For this review, take the finished solid that the model builds, in its own axes (mm). Face numbers are marked on the shaded views. Coordinates: 2 decimals unless noted, no trailing zeros. Write each question's results on one line, items separated by ' | '.
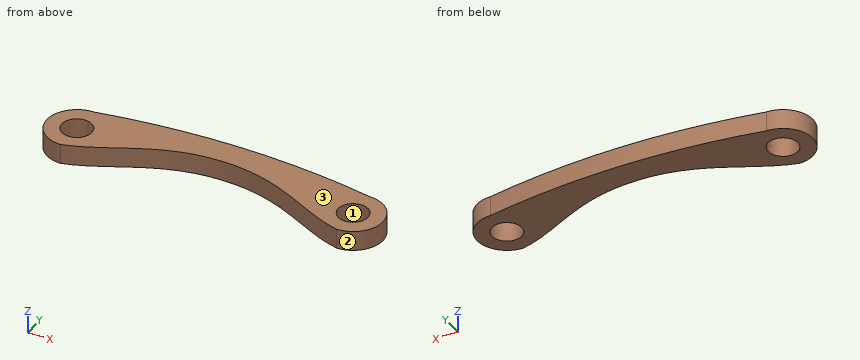
from build123d import *

# Parameters (mm, degrees)
SKETCH1_R           = 1.5
BOSS_EXTRUDE1_DEPTH = 2


with BuildPart() as part:
    # Sketch1 → Boss-Extrude1 (new body)
    with BuildSketch(Plane.XY):
        with BuildLine():
            ThreePointArc((-14, 3), (-17, 0), (-14, -3))
            add(Edge.make_bspline(
                [(-14, -3), (-10.110775288, -2.025488943), (-6.332313911, 1.681383892), (6.35903931, 1.579555666), (10.137986604, -2.11235599), (14, -3)],
                knots=[0, 0, 0, 0, 0.449202302, 0.549202302, 1, 1, 1, 1], degree=3))
            ThreePointArc((14, -3), (17, 0), (14, 3))
            add(Edge.make_bspline(
                [(-14, 3), (0, 5.7), (14, 3)],
                knots=[0, 0, 0, 1, 1, 1], degree=2))
        make_face()
        with Locations((-14, 0)):
            Circle(SKETCH1_R, mode=Mode.SUBTRACT)
        with Locations((14, 0)):
            Circle(SKETCH1_R, mode=Mode.SUBTRACT)
    extrude(amount=BOSS_EXTRUDE1_DEPTH)


solid = part.part
Q1. Wall thickness on line 1 along Y through (x, z) = (-14, 1.1); line 2 along X through (y, z) = (-0.5, 0.45); line 3 along Y through (x, z) = (-13, 1.7): over which ranges is each line inside the solid? List them lowest first. Write a range as from..to.
Results found:
line 1: -3..-1.5, 1.5..3 | line 2: -16.96..-15.41, -12.59..-8.26, 8.13..12.59, 15.41..16.96 | line 3: -2.7..-1.12, 1.12..3.19
Q2. For pin 1 (2 mm diameter, centred on x = 7.5, y = -2, fed in from -Z), flat-tipped, find the tip position at first contact; note if it passes through.
Results found:
pin 1: through
Q3. Take a section at A-A on z = 0.35. State how many separate pieces and enclosed holes the cut face has, plus the area to 3 significant figures.
Results found:
separate pieces: 1 | enclosed holes: 2 | area: 130 mm2
Q4. Mouldability with a two-part tool opening along Y and no side actions: class the marked faces 1, 2 and 3 as pulls with the +Y half, pulls with the -Y half, needs draft (parallel to the pull), parting line crosses it, or undercut.
Results found:
face 1: undercut | face 2: parting line crosses it | face 3: needs draft
